from build123d import *

# Parameters (mm, degrees)
BOSS_EXTRUDE1_DEPTH = 10


with BuildPart() as part:
    # Sketch1 → Boss-Extrude1 (new body)
    with BuildSketch(Plane(origin=(0, 0, 0), x_dir=(1, 0, 0), z_dir=(0, 1, 0))):
        Polygon((-31.591389498, 41.649056358), (-31.591389498, -24.112611576), (26.691500514, -24.112611576), (41.13327857, -5.544611218), (11.406624151, 17.576119997), (24.431058906, 28.088776811), (13.485895614, 41.649056358), align=None)
        Polygon((-23.854722682, 35.717611799), (9.155055732, 35.717611799), (15.022851217, 28.447830164), (3.172826817, 18.883097253), (-18.883097253, 18.883097253), (-10.365163505, 10.365163505), (3.172826817, 10.365163505), (23.338944894, -5.544611218), (13.255885856, -18.325191879), (-23.854722682, -18.325191879), align=None, mode=Mode.SUBTRACT)
    extrude(amount=BOSS_EXTRUDE1_DEPTH)


solid = part.part
For this review, take the finished solid that the model builds, in its own axes (mm). A direction names the side the tool comes from. Give positions to 0.01 mm unless a question says otherwise; leave off trailing zeros. Order: outer loops, then holes, each group sorted by start corner. A loop starts at its lowest first (then second) coordinate and runs counter-clockwise, first axis right, second up. Notation, with made-up numbers: (26.5, 26.5) - (43.5, 26.5) arc R20 ccw to (43.5, 55.5) - close; hole circle Ø3 at (10.25, 28). An arc over 180 degrees is marked (long way). Answer as a JSON object with one key per item and string values. Group by question number.
Item 1: Take a section at A-A on x = -14.5. Give the boundary of the cut face in (y, z), and give its area (3 significant figures).
Item 2: Take a section at C-C on x = -23. Give the boundary of the cut face in (y, z), and give its area (3 significant figures).
Item 3: Clearance check with flat-ended pins moving along their axes: pin 1 Ø10 at (x, z) = (31.5, -27) entering from +Y; pin 2 Ø6 at (y, z) = (8.5, 17) entering from +X. State where each tip first meets the part, or that it passes through.
Item 4: Machinability: for faces 1 (the flat face through (-8, 5, -18.883)), 2 (the flat face through (-31.591, 5, -9)), 3 (the flat face through (26.48, 4.93, -5.85)), which of the approach directions +Z, -Z, +X, -X, +Y, -Y give a long, thin tool a straight path to every point of the face, cutting with its end or side? Answer none if there is none.
Item 5: Wall thickness on line 1 along Z through (x, y) = (-7.5, 9.5); line 2 along Z through (x, y) = (6, 4.5); line 3 along Z through (x, y) = (-23, 3.5): over which ranges is each line inside the solid? List them lowest first.
Item 6: Draft analysis for pull direction Z (two halves, no side actions). For faces 4 (the flat face through (9.18, 4.93, -23.73)), 5 (the flat face through (-3, 5, 24.113)), 6 (the flat face through (-4, 0, -17)), 7 (the flat face through (-5, 5, 18.325)), state which applies: pulls with the +Z half, pulls with the -Z half, needs draft (parallel to the pull), parting line crosses it, or undercut.
Item 7: Take a section at B-B on y = 8.5. Give the boundary of the cut face in (x, z).
Item 8: Take a section at D-D on z = 1. Give the boundary of the cut face in (x, y).
Reported:
{
 "1": {"outline": "(0, -41.65) - (10, -41.65) - (10, -35.72) - (0, -35.72) - close; (0, -18.88) - (10, -18.88) - (10, -14.5) - (0, -14.5) - close; (0, 18.33) - (10, 18.33) - (10, 24.11) - (0, 24.11) - close", "area": "161 mm^2"},
 "2": {"outline": "(0, -41.65) - (10, -41.65) - (10, -35.72) - (0, -35.72) - close; (0, 18.33) - (10, 18.33) - (10, 24.11) - (0, 24.11) - close", "area": "117 mm^2"},
 "3": {"pin 1": "through", "pin 2": "x = 34.56"},
 "4": {"face 1": "+Y, -Y", "face 2": "+Z, -Z, -X, +Y, -Y", "face 3": "+X, +Y, -Y"},
 "5": {"line 1": "-41.65 to -35.72, -18.88 to -10.37, 18.33 to 24.11", "line 2": "-41.65 to -35.72, -21.17 to -8.13, 18.33 to 24.11", "line 3": "-41.65 to -35.72, 18.33 to 24.11"},
 "6": {"face 4": "undercut", "face 5": "pulls with the +Z half", "face 6": "needs draft", "face 7": "undercut"},
 "7": {"outline": "(-31.59, -41.65) - (13.49, -41.65) - (24.43, -28.09) - (11.41, -17.58) - (41.13, 5.54) - (26.69, 24.11) - (-31.59, 24.11) - close; hole (-23.85, -35.72) - (9.16, -35.72) - (15.02, -28.45) - (3.17, -18.88) - (-18.88, -18.88) - (-10.37, -10.37) - (3.17, -10.37) - (23.34, 5.54) - (13.26, 18.33) - (-23.85, 18.33) - close"},
 "8": {"outline": "(-31.59, 0) - (-23.85, 0) - (-23.85, 10) - (-31.59, 10) - close; (17.58, 0) - (35.29, 0) - (35.29, 10) - (17.58, 10) - close"}
}
